The figure shows three views and two pictorial views of one solid part (mm, origin at its lowest corner). Answer the questions. A direction names the side the tool comes from. Coordinates: 2 decimals unless noted, no trailing zeros. Write each loop counter-clockwise with the first axis right and the second up, starting at its lowest first coordinate (ties: lowest second). Pieces come first, ordered by that corner, then holes. Notation, with made-up numbers: M -14.75,70 L 22.25,70 A18 ccw 22.25,88 Z; hole C 7.25,71.25 d6. An arc over 180 degrees is marked long. Use CSV: the item, a comma, the result in double quotes.
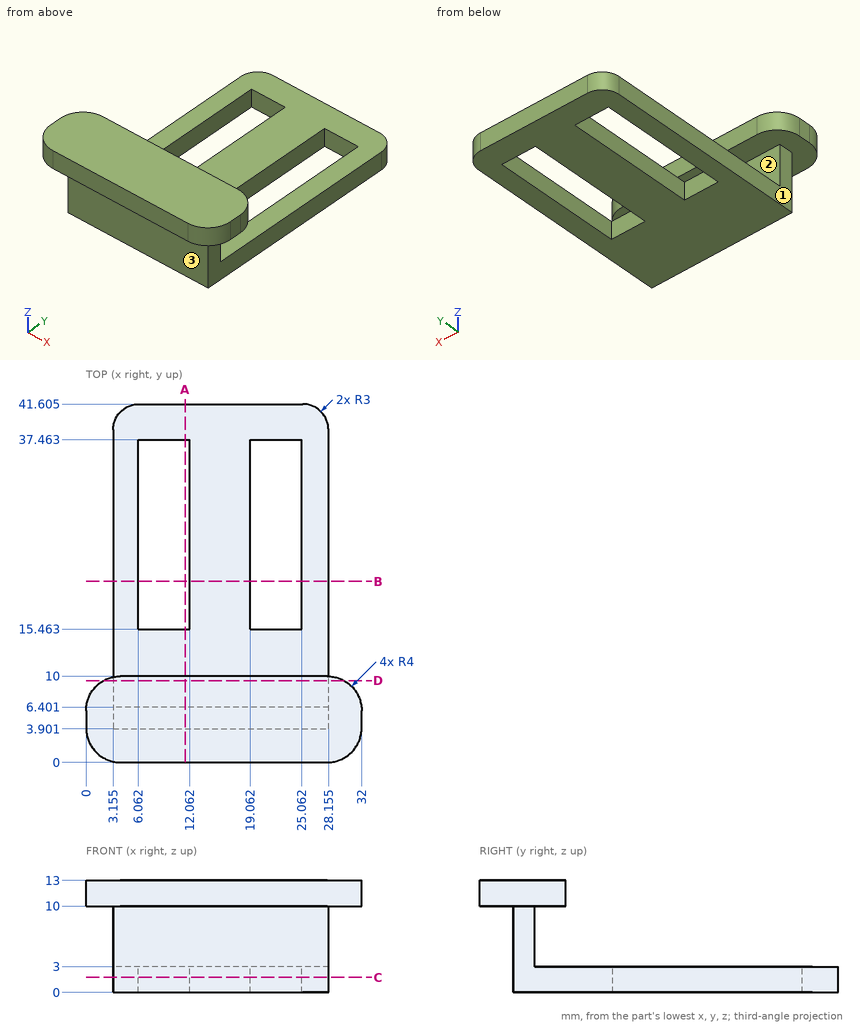
Item 1: The part is cut by section A-A (x = 11.5). Write down the section's boundary in (y, z) (1 decimal).
Answer:
outline,"M 0,10 L 3.9,10 L 3.9,0 L 15.5,0 L 15.5,3 L 6.4,3 L 6.4,10 L 10,10 L 10,13 L 0,13 Z; M 37.5,0 L 41.6,0 L 41.6,3 L 37.5,3 Z"
Item 2: A tool of negligible diameter and unlimited length cuts with its end or side. For the marked faces 1, 2 and 3, from which of +Z, -Z, +X, -X, +Y, -Y can it reach the whole face along a straight path? Write none if from no direction.
Answer:
face 1,"-Z, -X, +Y, -Y"
face 2,"+X, -X, +Y"
face 3,"-Z, +X, -X, -Y"
Item 3: The part is cut by section D-D (y = 9.5). Write down the section's boundary in (x, z) (1 decimal).
Answer:
outline,"M 2.1,10 L 29.9,10 L 29.9,13 L 2.1,13 Z; M 3.2,0 L 28.2,0 L 28.2,3 L 3.2,3 Z"
Item 4: Given pin 1 (2.5 mm diameter, centred on x = 13, z = 11, fed in from +Y); pin 2 (1 mm diameter, centred on x = 22, z = 9, fed in from -Y); pin 3 (0.9 mm diameter, centred on y = 31, z = 1.5, fed in from -X) (1 decimal), each flat-ended and moving along its own axis, determine where each tip first touches the part or whether it passes through.
Answer:
pin 1,"stops at y = 10"
pin 2,"stops at y = 3.9"
pin 3,"stops at x = 3.2"
Item 5: The part is cut by section C-C (z = 1.75). Write down the section's boundary in (x, y) (1 decimal), then the cut area to 3 significant figures.
Answer:
outline,"M 3.2,3.9 L 28.2,3.9 L 28.2,38.6 A3 ccw 25.2,41.6 L 6.2,41.6 A3 ccw 3.2,38.6 Z; hole M 6.1,15.5 L 12.1,15.5 L 12.1,37.5 L 6.1,37.5 Z; hole M 19.1,15.5 L 25.1,15.5 L 25.1,37.5 L 19.1,37.5 Z"
area,"675 mm2"
Item 6: Consider probe 1 along X at (y, z) = (20, 1.5) (1 decimal); probe 2 along Y at (x, z) = (12, 10.5); probe 3 along Z at (x, y) = (11.5, 14). Determine where each line is inside the solid, lowest interval first.
Answer:
probe 1,"x = 3.2 to 6.1, 12.1 to 19.1, 25.1 to 28.2"
probe 2,"y = 0 to 10"
probe 3,"z = 0 to 3"
Item 7: The part is cut by section B-B (y = 21). Write down the section's boundary in (x, z) (1 decimal), then the cut area to 3 significant figures.
Answer:
outline,"M 3.2,0 L 6.1,0 L 6.1,3 L 3.2,3 Z; M 12.1,0 L 19.1,0 L 19.1,3 L 12.1,3 Z; M 25.1,0 L 28.2,0 L 28.2,3 L 25.1,3 Z"
area,"39.0 mm2"
